For this review, take the finished solid that the model builds, in its own axes (mm). A direction names the side the tool comes from. Give positions to 0.01 mm unless a question says otherwise; leave off trailing zeros. Loops run counter-clockwise (first coordinate to the right, second up) from the corner with the lowest first, then second, coordinate; pieces in that order, holes last. Notation, with made-up numbers: (40, 56.5) -> (82, 56.5) arc R31 ccw to (82, 92.5) -> close; hole circle Ø7 at (9, 31.25). An arc over 180 degrees is marked (long way). Write each question's results on one line, items separated by ' | '. Start each with the question number.
```python
from build123d import *

# Parameters (mm, degrees)
F1_DEPTH = 12.5
F2_R     = 10
F3_R     = 10
F4_W     = 10
F4_H     = 10
F5_DEPTH = 6


with BuildPart() as f1:
    # F0 (on Top) → F1 (new body, symmetric)
    with BuildSketch(Plane.XY):
        Polygon((16.076079, 2.923578), (-13.923921, 2.923578), (-13.923921, -3.076422), (16.076079, -3.076422), (53.058334, 14.969733), (173.058334, 14.969733), (173.058334, 20.969733), (53.058334, 20.969733), align=None)
    extrude(amount=F1_DEPTH, both=True)

    # F2
    f2_edges = [f1.edges().sort_by_distance(p)[0] for p in [
        (-13.923921, -0.076422, 12.5),
    ]]
    fillet(f2_edges, radius=F2_R)

    # F3
    f3_edges = [f1.edges().sort_by_distance(p)[0] for p in [
        (-13.923921, -0.076422, -12.5),
        (173.058334, 17.969733, 12.5),
        (173.058334, 17.969733, -12.5),
    ]]
    fillet(f3_edges, radius=F3_R)

    # F4 (on face) → F5 (cut, through all)
    with BuildSketch(Plane(origin=(0, 2.923578, 0), x_dir=(-1, 0, 0), z_dir=(0, 1, 0))):
        Rectangle(F4_W, F4_H)
    extrude(amount=-F5_DEPTH, mode=Mode.SUBTRACT)


solid = f1.part
```
1. We need section C-C (z = 10.5). Write out the cut boundary in (x, y).
2. We need section D-D (x = 35.5). Write out the cut boundary in (y, z), plus the area to 3 significant figures.
3. Wall thickness on L1, parallel to Y at x = 62.5, z = -10; L2, parallel to X at y = 0, z = -1.75; L3, parallel to Y at x = 10.5, z = -9.25: over which ranges is each line inside the solid? List them lowest first.
4. For pin 1 Ø6.5 at (y, z) = (1, -1) entering from +X; pin 2 Ø8 at (x, z) = (78, -2) entering from -Y; pin 3 Ø8 at (y, z) = (11.5, -8.5) entering from -X, all flat-tipped, find the tip position at first contact; note any pin that passes through.
5. We need section A-A (z = -0.75). Write out the cut boundary in (x, y), plus the area to 3 significant figures.
6. We need section B-B (y = -1). Write out the cut boundary in (x, z).
7. Machinability: for faces 4 (the flat face through (112, 14.97, 0)), 5 (the flat face through (0, 0, -5)), 6 (the flat face through (114, 20.97, 0)), which of the approach directions +Z, -Z, +X, -X, +Y, -Y give a long, thin tool a straight path to every point of the face, cutting with its end or side? Answer none if there is none.
8. Draft analysis for pull direction Z (two halves, no side actions). For faces 1 (the flat face through (1.3, 2.924, -5.4)), 2 (the flat face through (79.2, 15.2, -12.5)), 3 (the flat face through (0, 0, 5)), state which applies: released by +Z, released by -Z, zero draft, split by the parting line, or undercut.
Response:
1) outline: (-9.92, -3.08) -> (16.08, -3.08) -> (53.06, 14.97) -> (169.06, 14.97) -> (169.06, 20.97) -> (53.06, 20.97) -> (16.08, 2.92) -> (-9.92, 2.92) -> close
2) outline: (6.4, -12.5) -> (12.4, -12.5) -> (12.4, 12.5) -> (6.4, 12.5) -> close | area: 150 mm2
3) L1: y = 14.97 to 20.97 | L2: x = -13.92 to -5, 5 to 22.38 | L3: y = -3.08 to 2.92
4) pin 1: stops at x = 31.09 | pin 2: stops at y = 14.97 | pin 3: stops at x = 25.45
5) outline: (-13.92, -3.08) -> (-5, -3.08) -> (-5, 2.92) -> (-13.92, 2.92) -> close; (5, -3.08) -> (16.08, -3.08) -> (53.06, 14.97) -> (173.06, 14.97) -> (173.06, 20.97) -> (53.06, 20.97) -> (16.08, 2.92) -> (5, 2.92) -> close | area: 1,060 mm2
6) outline: (-13.92, -2.5) arc R10 ccw to (-3.92, -12.5) -> (20.33, -12.5) -> (20.33, 12.5) -> (-3.92, 12.5) arc R10 ccw to (-13.92, 2.5) -> close; hole (-5, -5) -> (5, -5) -> (5, 5) -> (-5, 5) -> close
7) face 4: +Z, -Z, +X, -Y | face 5: +Y, -Y | face 6: +Z, -Z, +X, -X, +Y
8) face 1: zero draft | face 2: released by -Z | face 3: undercut
